Could you check a few things on this model? Use its own coordinates, in mm. Face numbers are marked on the shaded views. A direction names the side the tool comes from. Coordinates: 2 decimals unless noted, no trailing zeros. Loops run counter-clockwise (first coordinate to the right, second up) from the corner with the lowest first, then second, coordinate; pieces in that order, holes last. Notation, with made-up numbers: (-23.75, -4) - (17.25, -4) arc R29 cw to (17.25, 23) - close; hole circle Ø8 at (46, 49). An arc over 180 degrees is marked (long way). Put each result on its own line as item: value. Start each with the question number.
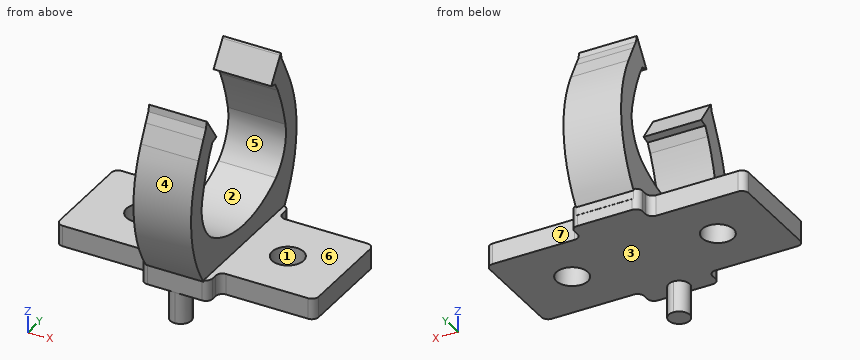
```python
from build123d import *

# Parameters (mm, degrees)
F0_R     = 2.9972
F0_R_2   = 3
F1_DEPTH = 4
F4_DEPTH = 5.5
F5_DEPTH = 5.5
F7_DEPTH = 6


with BuildPart() as f1:
    # F0 (on Top) → F1 (new body)
    with BuildSketch(Plane.XY):
        with BuildLine():
            Line((-25.6610898641, 24.5893044506), (-41.3210898641, 24.5893044506))
            ThreePointArc((-41.3210898641, 24.5893044506), (-42.2191154762, 24.2173300627), (-42.5910898641, 23.3193044506))
            Line((-42.5910898641, 23.3193044506), (-42.5910898641, 5.8593044506))
            ThreePointArc((-42.5910898641, 5.8593044506), (-42.2191154762, 4.9612788385), (-41.3210898641, 4.5893044506))
            Line((-41.3210898641, 4.5893044506), (-25.6610898641, 4.5893044506))
            ThreePointArc((-25.6610898641, 4.5893044506), (-24.763064252, 4.2173300627), (-24.3910898641, 3.3193044506))
            Line((-24.3910898641, 3.3193044506), (-24.3910898641, 2.2593044506))
            ThreePointArc((-24.3910898641, 2.2593044506), (-24.0191154762, 1.3612788385), (-23.1210898641, 0.9893044506))
            Line((-23.1210898641, 0.9893044506), (-17.8910898641, 0.9893044506))
            Line((-17.8910898641, 0.9893044506), (-17.8910898641, 28.1893044506))
            Line((-17.8910898641, 28.1893044506), (-23.1210898641, 28.1893044506))
            ThreePointArc((-23.1210898641, 28.1893044506), (-24.0191154762, 27.8173300627), (-24.3910898641, 26.9193044506))
            Line((-24.3910898641, 26.9193044506), (-24.3910898641, 25.8593044506))
            ThreePointArc((-24.3910898641, 25.8593044506), (-24.763064252, 24.9612788385), (-25.6610898641, 24.5893044506))
        make_face()
        with Locations((-31.7938898641, 14.5969044506)):
            Circle(F0_R, mode=Mode.SUBTRACT)
        with BuildLine():
            Line((-12.6610898641, 28.1893044506), (-17.8910898641, 28.1893044506))
            Line((-17.8910898641, 28.1893044506), (-17.8910898641, 0.9893044506))
            Line((-17.8910898641, 0.9893044506), (-12.6610898641, 0.9893044506))
            ThreePointArc((-12.6610898641, 0.9893044506), (-11.763064252, 1.3612788385), (-11.3910898641, 2.2593044506))
            Line((-11.3910898641, 2.2593044506), (-11.3910898641, 3.3193044506))
            ThreePointArc((-11.3910898641, 3.3193044506), (-11.0191154762, 4.2173300627), (-10.1210898641, 4.5893044506))
            Line((-10.1210898641, 4.5893044506), (5.5389101359, 4.5893044506))
            ThreePointArc((5.5389101359, 4.5893044506), (6.436935748, 4.9612788385), (6.8089101359, 5.8593044506))
            Line((6.8089101359, 5.8593044506), (6.8089101359, 23.3193044506))
            ThreePointArc((6.8089101359, 23.3193044506), (6.436935748, 24.2173300627), (5.5389101359, 24.5893044506))
            Line((5.5389101359, 24.5893044506), (-10.1210898641, 24.5893044506))
            ThreePointArc((-10.1210898641, 24.5893044506), (-11.0191154762, 24.9612788385), (-11.3910898641, 25.8593044506))
            Line((-11.3910898641, 25.8593044506), (-11.3910898641, 26.9193044506))
            ThreePointArc((-11.3910898641, 26.9193044506), (-11.763064252, 27.8173300627), (-12.6610898641, 28.1893044506))
        make_face()
        with Locations((-3.9910898641, 14.5893044506)):
            Circle(F0_R_2, mode=Mode.SUBTRACT)
    extrude(amount=F1_DEPTH)

    # F3 (on offset) → F4 (join)
    with BuildSketch(Plane.YZ.offset(-17.907)):
        with BuildLine():
            Line((1.0103175882, 3.6736566108), (1.0103175882, 2.094399018))
            Line((1.0103175882, 2.094399018), (14.6140140714, 2.094399018))
            Line((14.6140140714, 2.094399018), (14.6140140714, 7.5688682606))
            ThreePointArc((14.6140140714, 7.5688682606), (8.9162605334, 8.4182832346), (3.7140140714, 10.8926584944))
            ThreePointArc((3.7140140714, 10.8926584944), (0.9193465512, 14.8041987102), (0.5140140714, 19.594399018))
            ThreePointArc((0.5140140714, 19.594399018), (1.5880995617, 23.6670004727), (3.1097049359, 27.594399018))
            Line((3.1097049359, 27.594399018), (3.9924437818, 29.2461096572))
            Line((3.9924437818, 29.2461096572), (5.3628443275, 29.6174231917))
            Line((5.3628443275, 29.6174231917), (2.3336572567, 34.0493805554))
            Line((2.3336572567, 34.0493805554), (2.0878820214, 34.3491211534))
            Line((2.0878820214, 34.3491211534), (1.8287835856, 33.1069578199))
            Line((1.8287835856, 33.1069578199), (0.9140140714, 31.3994027674))
            Line((0.9140140714, 31.3994027674), (-0.6859859286, 28.1615126878))
            ThreePointArc((-0.6859859286, 28.1615126878), (-3.1482462474, 15.6882683861), (1.0103175882, 3.6736566108))
        make_face()
        with BuildLine():
            Line((14.6140140714, 7.5688682606), (14.6140140714, 2.094399018))
            Line((14.6140140714, 2.094399018), (28.2177105546, 2.094399018))
            Line((28.2177105546, 2.094399018), (28.2177105546, 3.6736566108))
            ThreePointArc((28.2177105546, 3.6736566108), (32.3762743902, 15.6882683861), (29.9140140714, 28.1615126878))
            Line((29.9140140714, 28.1615126878), (28.3140140714, 31.3994027674))
            Line((28.3140140714, 31.3994027674), (27.3992445572, 33.1069578199))
            Line((27.3992445572, 33.1069578199), (27.1401461214, 34.3491211534))
            Line((27.1401461214, 34.3491211534), (26.8943708861, 34.0493805554))
            Line((26.8943708861, 34.0493805554), (23.8651838154, 29.6174231917))
            Line((23.8651838154, 29.6174231917), (25.2355843611, 29.2461096572))
            Line((25.2355843611, 29.2461096572), (26.1183232069, 27.594399018))
            ThreePointArc((26.1183232069, 27.594399018), (27.6399285811, 23.6670004727), (28.7140140714, 19.594399018))
            ThreePointArc((28.7140140714, 19.594399018), (28.3086815916, 14.8041987102), (25.5140140714, 10.8926584944))
            ThreePointArc((25.5140140714, 10.8926584944), (20.3117676094, 8.4182832346), (14.6140140714, 7.5688682606))
        make_face()
    extrude(amount=F4_DEPTH)

    # F5 (add): a face of the model
    f5_faces = [f1.faces().sort_by_distance(p)[0] for p in [
        (-17.907, 0.5449617654, 29.5675053748),
    ]]
    extrude(f5_faces, amount=F5_DEPTH)

    # F6 (on face) → F7 (join)
    with BuildSketch(Plane.XY):
        with BuildLine():
            ThreePointArc((-17.8910898641, 0.9894171115), (-16.4631735111, 1.5676054433), (-15.8698617965, 2.9893044506))
            ThreePointArc((-15.8698617965, 2.9893044506), (-16.4631735111, 4.411003458), (-17.8910898641, 4.9891917898))
            Line((-17.8910898641, 4.9891917898), (-17.8910898641, 0.9894171115))
        make_face()
        with BuildLine():
            Line((-17.8910898641, 0.9894171115), (-17.8910898641, 4.9891917898))
            ThreePointArc((-17.8910898641, 4.9891917898), (-19.8698617965, 2.9893044506), (-17.8910898641, 0.9894171115))
        make_face()
    extrude(amount=-F7_DEPTH)


solid = f1.part
```
(1) I need wall thicknesses on L1, parallel to Z at x = -19, y = 3.5; L2, parallel to Y at x = -15, z = 28.5; L3, parallel to Z at x = -12, y = 3. Which ranges of each line are inside material? Lowest first, please. Write a range as [from, to].
(2) I want a section at A-A on z = 9. List the corners of the cut face in (x, y) for me, and give its area (3 significant figures).
(3) Which directions (+Z, -Z, +X, -X, +Y, -Y) give clear straight access to the entire face, cutting with the end or side of a thin tool? Please do the marked faces 5, 6 and 7.
(4) I want a section at C-C on x = -34. List the corners of the cut face in (y, z) for me.
(5) For pin 1 Ø16 at (y, z) = (9, 14.5) entering from -X; pin 2 Ø1 at (x, y) = (-22, 19.5) entering from -Z; pin 3 Ø1 at (x, z) = (-1, -1.5) entering from +Y; pin 4 Ø1 at (x, y) = (-19, 29) entering from -Z, each with a flat end and sliding along its axis, tell me the tip position at first contact or that it passes through.
(6) If we mould it in two halves opening along Y, with no side actions, what happens to the marked faces 1, 2, 3 and 4? For each: pulls with the +Y half, pulls with the -Y half, needs draft (parallel to the pull), parting line crosses it, or undercut.
(7) I want a section at B-B on y = 16.5. List the corners of the cut face in (x, z) for me, and give its area (3 significant figures).
Answer sheet:
1. L1: z = [-6, 11.07], [28.32, 32.34]
1. L2: y = [-0.52, 3.59], [25.63, 29.75]
1. L3: z = [0, 4]
2. outline: (-23.41, -1.72) - (-12.41, -1.72) - (-12.41, 7.27) - (-23.41, 7.27) - close; (-23.41, 21.95) - (-12.41, 21.95) - (-12.41, 30.95) - (-23.41, 30.95) - close
2. area: 198 mm^2
3. face 5: +X, -X
3. face 6: +Z, +X, +Y, -Y
3. face 7: +Z, -Z, +X, +Y
4. outline: (4.59, 0) - (12.57, 0) - (12.57, 4) - (4.59, 4) - close; (16.63, 0) - (24.59, 0) - (24.59, 4) - (16.63, 4) - close
5. pin 1: stops at x = -23.41
5. pin 2: stops at z = 0
5. pin 3: passes through
5. pin 4: stops at z = 4.1
6. face 1: undercut
6. face 2: undercut
6. face 3: needs draft
6. face 4: pulls with the -Y half
7. outline: (-42.59, 0) - (-34.11, 0) - (-34.11, 4) - (-42.59, 4) - close; (-29.48, 0) - (-6.3, 0) - (-6.3, 4) - (-12.41, 4) - (-12.41, 7.66) - (-23.41, 7.66) - (-23.41, 4) - (-29.48, 4) - close; (-1.68, 0) - (6.81, 0) - (6.81, 4) - (-1.68, 4) - close
7. area: 201 mm^2
